```python
from build123d import *

# Parameters (mm, degrees)
BOSS_EXTRUDE1_DEPTH = 12
CUT_EXTRUDE1_DEPTH  = 12


with BuildPart() as part:
    # Sketch1 → Boss-Extrude1 (new body)
    with BuildSketch(Plane.XY):
        with BuildLine():
            Line((-45.137913667, 106.817655073), (-56.782603372, 86.648460865))
            ThreePointArc((-56.782603372, 86.648460865), (-76.884990379, 71.629544832), (-83.401578598, 47.397172266))
            ThreePointArc((-83.401578598, 47.397172266), (-83.862908864, 41.49589237), (-86.031372169, 35.98810725))
            Line((-86.031372169, 35.98810725), (-94.257114543, 21.740703527))
            Line((-94.257114543, 21.740703527), (-73.496897515, 21.740703527))
            Line((-73.496897515, 21.740703527), (-73.496897515, 50.099687376))
            ThreePointArc((-73.496897515, 50.099687376), (-45.137913667, 78.458671224), (-16.778929818, 50.099687376))
            Line((-16.778929818, 50.099687376), (-16.778929818, 21.740703527))
            Line((-16.778929818, 21.740703527), (3.98128721, 21.740703527))
            Line((3.98128721, 21.740703527), (-4.244455165, 35.98810725))
            ThreePointArc((-4.244455165, 35.98810725), (-6.412918469, 41.49589237), (-6.874248735, 47.397172266))
            ThreePointArc((-6.874248735, 47.397172266), (-13.390836954, 71.629544832), (-33.493223961, 86.648460865))
            Line((-33.493223961, 86.648460865), (-45.137913667, 106.817655073))
        make_face()
    extrude(amount=BOSS_EXTRUDE1_DEPTH)

    # Sketch2 → Cut-Extrude1 (cut)
    with BuildSketch(Plane.XY.offset(12)):
        Polygon((-52.018755525, 94.899687376), (-38.257071808, 94.899687376), (-45.137913667, 106.817655073), align=None)
        Polygon((-80.495430827, 21.740703527), (-87.376272685, 33.658671224), (-94.257114543, 21.740703527), align=None)
        Polygon((-2.899554648, 33.658671224), (-9.780396506, 21.740703527), (3.98128721, 21.740703527), align=None)
    extrude(amount=-CUT_EXTRUDE1_DEPTH, mode=Mode.SUBTRACT)


solid = part.part
```
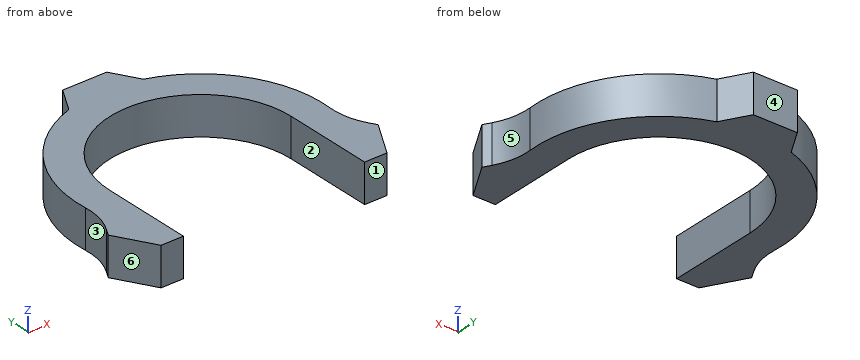
Can you work these out from the model? Positions are in its coordinate system, mm. Face numbers are marked on the shaded views. A direction names the side the tool comes from. Coordinates: 2 decimals unless noted, no trailing zeros. Order: outer loops, then holes, each group sorted by start corner. A loop starts at its lowest first (then second) coordinate and runs counter-clockwise, first axis right, second up.
1. If we section it at B-B (z = 4): Please give me the cut outline in (x, y), then the cut area to 3 significant figures.
2. Thinking about a two-plate mould opening in Y: for the marked faces 3, 4, 5 and 6, which applies, +Y half, -Y half, draft (parallel to the pull), parting line (faces both ways), or undercut?
3. For the marked faces 1 and 2, which set-ups out of +Z, -Z, +X, -X, +Y, -Y let a thin tool reach every point of the face, with its end or its side?
4. If we section it at C-C (y = 29): Please give me the cut outline in (x, z).
5. If we section it at D-D (x = -69.5): Please give me the cut outline in (y, z).
6. I need wall thicknesses on line 1 (X direction, y = 43.5, z = 10); line 2 (X direction, y = 47.5, z = 9.5); line 3 (X direction, y = 81.5, z = 10.5). Which ranges of each line are inside material? Lowest first, please.
7. If we section it at A-A (y = 75.5): Please give me the cut outline in (x, z), then the cut area to 3 significant figures.
8. I'm going to push flat-ended pins straight in: pin 1 (4 mm diameter, centred on y = 65, z = 6, fed in from -X); pin 2 (6 mm diameter, centred on y = 38, z = 8.5, fed in from +X); pin 3 (6 mm diameter, centred on y = 39.5, z = 5.5, fed in from -X). Where does each tip first touch, or does it pass through?
Entries:
1. outline: (-87.38, 33.66) - (-80.5, 21.74) - (-73.5, 21.74) - (-73.5, 50.1) arc R28.36 cw to (-16.78, 50.1) - (-16.78, 21.74) - (-9.78, 21.74) - (-2.9, 33.66) - (-4.24, 35.99) arc R20 cw to (-6.87, 47.4) arc R38.36 ccw to (-33.49, 86.65) - (-38.26, 94.9) - (-52.02, 94.9) - (-56.78, 86.65) arc R38.36 ccw to (-83.4, 47.4) arc R20 cw to (-86.03, 35.99) - close
1. area: 1,780 mm2
2. face 3: undercut
2. face 4: +Y half
2. face 5: undercut
2. face 6: -Y half
3. face 1: +Z, -Z, +X, -X, -Y
3. face 2: +Z, -Z, -Y
4. outline: (-84.69, 0) - (-73.5, 0) - (-73.5, 12) - (-84.69, 12) - close; (-16.78, 0) - (-5.59, 0) - (-5.59, 12) - (-16.78, 12) - close
5. outline: (64.62, 0) - (79.73, 0) - (79.73, 12) - (64.62, 12) - close
6. line 1: x = -83.51 to -73.5, -16.78 to -6.77
6. line 2: x = -83.41 to -73.5, -16.78 to -6.87
6. line 3: x = -67.17 to -23.11
7. outline: (-73.88, 0) - (-57.75, 0) - (-57.75, 12) - (-73.88, 12) - close; (-32.53, 0) - (-16.39, 0) - (-16.39, 12) - (-32.53, 12) - close
7. area: 387 mm2
8. pin 1: stops at x = -81.26
8. pin 2: stops at x = -3.67
8. pin 3: stops at x = -85.75
